Geometry check sheet. Reference: the model listing, model coordinates, mm. A direction names the side the tool comes from. Round coordinates to 2 decimals unless told otherwise and drop trailing zeros. Order: outer loops, then holes, each group sorted by start corner. A loop starts at its lowest first (then second) coordinate and runs counter-clockwise, first axis right, second up.
(1) Set-up check for faces 1 (the face through (6, -1, 3)), 2 (the face through (16, -1, 18)), 3 (the face through (11.106, -0.7, 2.156)): record each of +Z, -Z, +X, -X, +Y, -Y from which the full face is reachable in a straight line by a thin tool's end or side.
(2) Cross-section at A-A on z = 22. Enter the section's corners in (x, y).
(3) Gauge pin test, flat ends, axial feed: P1, Ø2, axis at y = 21, z = 3.5, coming from the -X side; P2, Ø2, axis at y = 16.5, z = 3, coming from the +X side. Record the tip position at first contact, or that the pin passes through.
(4) Thickness scan on L1, parallel to X at y = -28.5, z = 9; L2, parallel to Z at x = 2, y = -11; L3, parallel to Z at x = 9, y = -27. Record the ranges inside material, lowest first.
(5) Draft check along X on faces 4 (the face through (-0.1, 50, 28.4)), 5 (the face through (-10.964, -0.7, 2.118)), 6 (the face through (-16, -1, 18)). Enter one of: pulls with the +X half, pulls with the -X half, needs draft (parallel to the pull), parting line crosses it, or undercut.
(6) Cross-section at B-B on y = -18. Enter the section's corners in (x, z), and give its area (3 significant figures).
(7) Cross-section at C-C on x = -9.5. Enter the section's corners in (y, z), and give its area (3 significant figures).
(8) Cross-section at D-D on x = -4.5. Enter the section's corners in (y, z), and give its area (3 significant figures).
from build123d import *

# Parameters (mm, degrees)
F1_DEPTH = 50


with BuildPart() as f1:
    # F0 (on Front) → F1 (new body, symmetric)
    with BuildSketch(Plane.XZ):
        with BuildLine():
            Line((16, 30), (-16, 30))
            Line((-16, 30), (-16, 6))
            ThreePointArc((-16, 6), (-12.4494897428, 0.5227744249), (-6, 1.527864045))
            Line((-6, 1.527864045), (-6, 4))
            Line((-6, 4), (-6.5358986055, 4))
            ThreePointArc((-6.5358986055, 4), (-11.0352761842, 2.1362968937), (-13.9999998089, 6))
            Line((-13.9999998089, 6), (-13.9999998089, 27.9999998089))
            Line((-13.9999998089, 27.9999998089), (13.9999998089, 27.9999998089))
            Line((13.9999998089, 27.9999998089), (13.9999998089, 6))
            ThreePointArc((13.9999998089, 6), (11.0352761842, 2.1362968937), (6.5358986055, 4))
            Line((6.5358986055, 4), (6, 4))
            Line((6, 4), (6, 1.527864045))
            ThreePointArc((6, 1.527864045), (12.4494897428, 0.5227744249), (16, 6))
            Line((16, 6), (16, 30))
        make_face()
    extrude(amount=F1_DEPTH, both=True)


solid = f1.part
Found:
1. face 1: -Z, +Y, -Y
1. face 2: +Z, -Z, +X, +Y, -Y
1. face 3: +Y, -Y
2. outline: (-16, -50) - (-14, -50) - (-14, 50) - (-16, 50) - close; (14, -50) - (16, -50) - (16, 50) - (14, 50) - close
3. P1: stops at x = -15.81
3. P2: stops at x = 15.66
4. L1: x = -16 to -14, 14 to 16
4. L2: z = 28 to 30
4. L3: z = 0.08 to 2.13, 28 to 30
5. face 4: needs draft
5. face 5: undercut
5. face 6: pulls with the -X half
6. outline: (-16, 6) arc R6 ccw to (-6, 1.53) - (-6, 4) - (-6.54, 4) arc R4 cw to (-14, 6) - (-14, 28) - (14, 28) - (14, 6) arc R4 cw to (6.54, 4) - (6, 4) - (6, 1.53) arc R6 ccw to (16, 6) - (16, 30) - (-16, 30) - close
6. area: 202 mm2
7. outline: (-50, 0.02) - (50, 0.02) - (50, 2.03) - (-50, 2.03) - close; (-50, 28) - (50, 28) - (50, 30) - (-50, 30) - close
7. area: 401 mm2
8. outline: (-50, 28) - (50, 28) - (50, 30) - (-50, 30) - close
8. area: 200 mm2
